```python
from build123d import *

# Parameters (mm, degrees)
F0_W      = 30
F0_H      = 14
F1_DEPTH  = 10
F2_W      = 10.5
F2_H      = 5.7
F3_DEPTH  = 25
F4_R      = 4
F5_R      = 2
F6_DEPTH  = 25
F8_DEPTH  = 5
F10_DEPTH = 12
F11_R     = 0.7
F12_R     = 1
F13_R     = 2.5
F14_DEPTH = 15


with BuildPart() as f1:
    # F0 (on Top) → F1 (new body)
    with BuildSketch(Plane.XY):
        Rectangle(F0_W, F0_H)
    extrude(amount=F1_DEPTH)

    # F2 (on face) → F3 (cut)
    with BuildSketch(Plane.XY.offset(10)):
        with Locations((-9.75, -4.15)):
            Rectangle(F2_W, F2_H)
        with Locations((-9.75, 4.15)):
            Rectangle(F2_W, F2_H)
    extrude(amount=-F3_DEPTH, mode=Mode.SUBTRACT)

    # F4
    f4_edges = [f1.edges().sort_by_distance(p)[0] for p in [
        (-15, 0, 10),
        (-15, 0, 0),
        (-4.5, -4.15, 10),
        (-4.5, -4.15, 0),
        (-4.5, 4.15, 0),
        (-4.5, 4.15, 10),
    ]]
    fillet(f4_edges, radius=F4_R)

    # F5 (on face) → F6 (cut)
    with BuildSketch(Plane.XZ.offset(1.3)):
        with Locations((-11, 5)):
            Circle(F5_R)
    extrude(amount=-F6_DEPTH, mode=Mode.SUBTRACT)

    # F7 (on face) → F8 (join)
    with BuildSketch(Plane.YZ.offset(15)):
        with BuildLine():
            ThreePointArc((0, 0), (3.5355339059, 1.4644660941), (5, 5))
            ThreePointArc((5, 5), (3.5355339059, 8.5355339059), (0, 10))
            ThreePointArc((0, 10), (-5, 5), (0, 0))
        make_face()
    extrude(amount=F8_DEPTH)

    # F9 (on face) → F10 (cut)
    with BuildSketch(Plane.XY.offset(10)):
        Polygon((10, -5), (9.9985566437, 5), (3.9985566437, 5), (3.9985566437, -5), align=None)
    extrude(amount=-F10_DEPTH, mode=Mode.SUBTRACT)

    # F11
    f11_edges = [f1.edges().sort_by_distance(p)[0] for p in [
        (-5.75, -1.3, 10),
        (-5.75, -1.3, 0),
        (-13.828427, -1.3, 1.171573),
        (-15, -1.3, 5),
        (-13.828427, -1.3, 8.828427),
        (-5.75, 1.3, 0),
        (-13.828427, 1.3, 1.171573),
        (-15, 1.3, 5),
        (-13.828427, 1.3, 8.828427),
        (-5.75, 1.3, 10),
    ]]
    fillet(f11_edges, radius=F11_R)

    # F12
    f12_edges = [f1.edges().sort_by_distance(p)[0] for p in [
        (7.25, -7, 10),
        (-3.328427, -7, 1.171573),
        (-4.5, -7, 5),
        (-3.328427, -7, 8.828427),
        (7.25, 7, 10),
    ]]
    fillet(f12_edges, radius=F12_R)

    # F13 (on face) → F14 (cut)
    with BuildSketch(Plane.YZ.offset(20)):
        with Locations((0, 5)):
            Circle(F13_R)
    extrude(amount=-F14_DEPTH, mode=Mode.SUBTRACT)


solid = f1.part
```
Geometry: final body of the model. Coordinates: model frame, mm. A direction names the side the tool comes from. Give positions to 0.01 mm unless a question says otherwise; leave off trailing zeros. Order: outer loops, then holes, each group sorted by start corner. A loop starts at its lowest first (then second) coordinate and runs counter-clockwise, first axis right, second up. Notation, with made-up numbers: M 36,13.25 L 44,13.25 A17 ccw 44,23.25 Z; hole C 3,-4.5 d1. An arc over 180 degrees is marked long. Answer as CSV lines item,"result". Start each with the question number.
1) Cut plane D-D (x = -8). Output: boundary loops of the cut face in (y, z), then the cut area to 3 significant figures.
2) Set-up query: faces 1 (the cylindrical face through (-3.297, 3.338, 8.859)), 2 (the cylindrical face through (-3.297, -3.262, 1.141)), 3 (the flat face through (7, 5, 5)), 4 (the cylindrical face through (15.07, 1.34, 7.11)), 5 (the flat face through (-4.5, 4, 5)). Return all of +Z, -Z, +X, -X, +Y, -Y with unobstructed straight access to the full face (end or side cutting, diameter ignored); none if empty.
3) Mould query, pull axis Y, two halves, no side actions, for faces 6 (the flat face through (20, 2, 3)), 7 (the cylindrical face through (7.358, -6.699, 9.715)), 8 (the flat face through (3.999, 0, 5)). Classes: +Y half, -Y half, draft (parallel to the pull), parting line (faces both ways), or undercut.
4) Cut plane B-B (x = 8). Output: boundary loops of the cut face in (y, z), then the cut area to 3 significant figures.
5) Cut plane A-A (x = 14). Output: boundary loops of the cut face in (y, z), then the cut area to 3 significant figures.
6) Line query: line 1 (X direction, y = -3.25, z = 5); line 2 (Y direction, x = 17, z = 5); line 3 (Y direction, x = 14, z = 5). Output: solid intervals per line, ascending. Write a range as from..to.
7) First-contact query: P1, Ø1, axis at y = 1.5, z = 4.5, coming from the +X side; P2, Ø2, axis at y = 3, z = 4.5, coming from the -X side; P3, Ø8, axis at x = -7, y = 5, coming from the +Z side. Flat tips, straight axial feed; report the tip coordinate or a pass-through.
8) Cut plane C-C (y = 4). Output: boundary loops of the cut face in (x, z), then the cut area to 3 significant figures.
Findings below:
1,outline,"M -1.3,0.7 A0.7 ccw -0.6,0 L 0.6,0 A0.7 ccw 1.3,0.7 L 1.3,9.3 A0.7 ccw 0.6,10 L -0.6,10 A0.7 ccw -1.3,9.3 Z"
1,area,"25.6 mm²"
2,face 1,"+Z, -X, +Y"
2,face 2,"-Z, -X, -Y"
2,face 3,"+Z, -Z"
2,face 4,"+X"
2,face 5,"+Z, -Z, -X, +Y"
3,face 6,"draft"
3,face 7,"-Y half"
3,face 8,"undercut"
4,outline,"M -7,1 A1 ccw -6,0 L -5,0 L -5,10 L -6,10 A1 ccw -7,9 Z; M 5,0 L 6,0 A1 ccw 7,1 L 7,9 A1 ccw 6,10 L 5,10 Z"
4,area,"39.1 mm²"
5,outline,"M -7,1 A1 ccw -6,0 L 6,0 A1 ccw 7,1 L 7,9 A1 ccw 6,10 L -6,10 A1 ccw -7,9 Z; hole C 0,5 d5"
5,area,"120 mm²"
6,line 1,"x = -4.5..4, 10..20"
6,line 2,"y = -5..-2.5, 2.5..5"
6,line 3,"y = -7..-2.5, 2.5..7"
7,P1,"stops at x = 4"
7,P2,"stops at x = -4.5"
7,P3,"stops at z = 9.87"
8,outline,"M -4.5,4 A4 ccw -0.5,0 L 4,0 L 4,10 L -0.5,10 A4 ccw -4.5,6 Z; M 10,0 L 15,0 L 15,2 L 20,2 L 20,8 L 15,8 L 15,10 L 10,10 Z"
8,area,"158 mm²"
